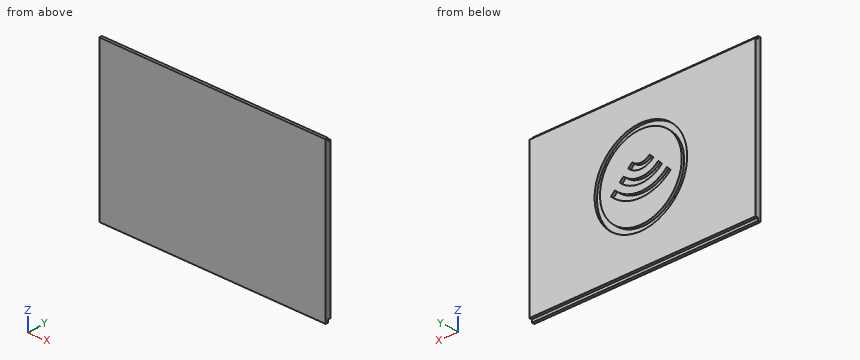
```python
from build123d import *

# Parameters (mm, degrees)
SKIZZE1_W                       = 83
SKIZZE1_H                       = 58
AUFSATZ_LINEAR_AUSTRAGEN1_DEPTH = 2
SKIZZE2_W                       = 83
SKIZZE2_H                       = 1
SCHNITT_LINEAR_AUSTRAGEN1_DEPTH = 1
SKIZZE3_R                       = 17
SKIZZE3_R_2                     = 15
SCHNITT_LINEAR_AUSTRAGEN2_DEPTH = 1


with BuildPart() as part:
    # Skizze1 → Aufsatz-Linear austragen1 (new body)
    with BuildSketch(Plane(origin=(0, 0, 0), x_dir=(1, 0, 0), z_dir=(0, 1, 0))):
        with Locations((41.5, 29)):
            Rectangle(SKIZZE1_W, SKIZZE1_H)
    extrude(amount=AUFSATZ_LINEAR_AUSTRAGEN1_DEPTH)

    # Skizze2 → Schnitt-Linear austragen1 (cut)
    with BuildSketch(Plane(origin=(0, 2, 0), x_dir=(1, 0, 0), z_dir=(0, 1, 0))):
        with Locations((41.5, 57.5)):
            Rectangle(SKIZZE2_W, SKIZZE2_H)
        with Locations((41.5, 0.5)):
            Rectangle(SKIZZE2_W, SKIZZE2_H)
    extrude(amount=-SCHNITT_LINEAR_AUSTRAGEN1_DEPTH, mode=Mode.SUBTRACT)

    # Skizze3 → Schnitt-Linear austragen2 (cut)
    with BuildSketch(Plane(origin=(0, 2, 0), x_dir=(1, 0, 0), z_dir=(0, 1, 0))):
        with Locations((42.119824852, 28.44050911)):
            Circle(SKIZZE3_R)
        with Locations((42.119824852, 28.44050911)):
            Circle(SKIZZE3_R_2, mode=Mode.SUBTRACT)
        with BuildLine():
            ThreePointArc((31.159669744, 30.400664218), (42.119824852, 34.94050911), (53.079979961, 30.400664218))
            Line((53.079979961, 30.400664218), (51.665766398, 28.986450656))
            ThreePointArc((51.665766398, 28.986450656), (42.119824852, 32.94050911), (32.573883306, 28.986450656))
            Line((32.573883306, 28.986450656), (31.159669744, 30.400664218))
        make_face()
        with BuildLine():
            Line((35.755863822, 25.80447014), (34.341650259, 27.218683703))
            ThreePointArc((34.341650259, 27.218683703), (42.119824852, 30.44050911), (49.897999445, 27.218683703))
            Line((49.897999445, 27.218683703), (48.483785883, 25.80447014))
            ThreePointArc((48.483785883, 25.80447014), (42.119824852, 28.44050911), (35.755863822, 25.80447014))
        make_face()
        with BuildLine():
            Line((38.937844337, 22.622489625), (37.523630775, 24.036703187))
            ThreePointArc((37.523630775, 24.036703187), (42.119824852, 25.94050911), (46.71601893, 24.036703187))
            Line((46.71601893, 24.036703187), (45.301805368, 22.622489625))
            ThreePointArc((45.301805368, 22.622489625), (42.119824852, 23.94050911), (38.937844337, 22.622489625))
        make_face()
    extrude(amount=-SCHNITT_LINEAR_AUSTRAGEN2_DEPTH, mode=Mode.SUBTRACT)


solid = part.part
```
Build history of the part. All positions in model axes, mm. Coordinates: 2 decimals unless noted, no trailing zeros. Write each loop counter-clockwise with the first axis right and the second up, starting at its lowest first coordinate (ties: lowest second). Pieces come first, ordered by that corner, then holes.
1. Band-saw the part on D-D, the plane z = -18. Give the cut face in (x, y), and give its area (3 significant figures).
Answer block:
outline: (0, 0) - (83, 0) - (83, 2) - (55.54, 2) - (55.54, 1) - (52.89, 1) - (52.89, 2) - (31.35, 2) - (31.35, 1) - (28.7, 1) - (28.7, 2) - (0, 2) - close
area: 161 mm2
2. Band-saw the part on B-B, the plane x = 10. Give the cut face in (y, z).
Answer block:
outline: (0, -58) - (1, -58) - (1, -57) - (2, -57) - (2, -1) - (1, -1) - (1, 0) - (0, 0) - close
3. Drop flat-ended pins along their axis: pin 1 (0.5 mm diameter, centred on x = 26.5, z = -0.5, fed in from +Y); pin 2 (0.5 mm diameter, centred on x = 30, y = 1.5, fed in from +Z). Give the stop position or say it passes through.
Answer block:
pin 1: stops at y = 1
pin 2: stops at z = -1
4. Band-saw the part on A-A, the plane y = 1.4. Give the cut face in (x, z), and give its area (3 significant figures).
Answer block:
outline: (0, -57) - (83, -57) - (83, -1) - (0, -1) - close; circle Ø30 at (42.12, -28.44); hole circle Ø34 at (42.12, -28.44); hole (31.16, -30.4) arc R15.5 ccw to (53.08, -30.4) - (51.67, -28.99) arc R13.5 cw to (32.57, -28.99) - close; hole (34.34, -27.22) arc R11 ccw to (49.9, -27.22) - (48.48, -25.8) arc R9 cw to (35.76, -25.8) - close; hole (37.52, -24.04) arc R6.5 ccw to (46.72, -24.04) - (45.3, -22.62) arc R4.5 cw to (38.94, -22.62) - close
area: 4,350 mm2
5. Band-saw the part on C-C, the plane z = -34. Give the cut face in (x, y).
Answer block:
outline: (0, 0) - (83, 0) - (83, 2) - (58.19, 2) - (58.19, 1) - (56.05, 1) - (56.05, 2) - (47.44, 2) - (47.44, 1) - (36.8, 1) - (36.8, 2) - (28.19, 2) - (28.19, 1) - (26.05, 1) - (26.05, 2) - (0, 2) - close
6. Drill centre lines: probe 1 along X at (y, z) = (1.15, -31.5); probe 2 along Z at (x, y) = (40.5, 1.55); probe 3 along X at (y, z) = (1.55, -27.5). Where is each one in solid material? Low to high.
Answer block:
probe 1: x = 0 to 25.4, 27.44 to 32.38, 36.05 to 48.19, 51.86 to 56.8, 58.84 to 83
probe 2: z = -57 to -45.36, -43.35 to -34.86, -32.84 to -30.32, -28.29 to -25.74, -23.64 to -13.53, -11.52 to -1
probe 3: x = 0 to 25.15, 27.15 to 34.63, 38.11 to 46.13, 49.61 to 57.09, 59.09 to 83
